CAD build for the part. Positions are in the model's coordinates, mm. Face numbers are marked on the shaded views. A direction names the side the tool comes from. Coordinates: 2 decimals unless noted, no trailing zeros. Write each loop counter-clockwise with the first axis right and the second up, starting at its lowest first coordinate (ties: lowest second). Pieces come first, ordered by that corner, then holes. Notation, with made-up numbers: (32, -17) -> (37, -17) arc R31 ccw to (37, 12) -> close; hole circle Ø4 at (81, 8). An arc over 180 degrees is marked (long way). Answer as CSV lines item,"result".
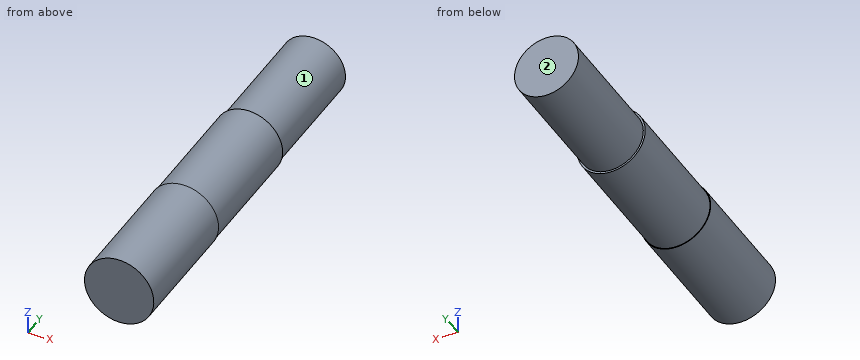
```python
from build123d import *

# Parameters (mm, degrees)
SKETCH1_R           = 4.7625
BOSS_EXTRUDE1_DEPTH = 38.1
SKETCH2_R           = 5.832464333
SKETCH2_R_2         = 3.3
CUT_EXTRUDE1_DEPTH  = 12.7
SKETCH3_R           = 5.346562202
SKETCH3_R_2         = 3.5
CUT_EXTRUDE2_DEPTH  = 12.7
SKETCH4_R           = 4.91764208
SKETCH4_R_2         = 3.571875
CUT_EXTRUDE3_DEPTH  = 12.7


with BuildPart() as part:
    # Sketch1 → Boss-Extrude1 (new body)
    with BuildSketch(Plane(origin=(0, 0, 0), x_dir=(1, 0, 0), z_dir=(0, 1, 0))):
        with Locations(Location((0, 0, 0), (0, 0, 90))):
            Circle(SKETCH1_R)
    extrude(amount=BOSS_EXTRUDE1_DEPTH)

    # Sketch2 → Cut-Extrude1 (cut)
    with BuildSketch(Plane(origin=(0, 38.1, 0), x_dir=(1, 0, 0), z_dir=(0, 1, 0))):
        Circle(SKETCH2_R)
        with Locations(Location((0, 0, 0), (0, 0, 270))):
            Circle(SKETCH2_R_2, mode=Mode.SUBTRACT)
    extrude(amount=-CUT_EXTRUDE1_DEPTH, mode=Mode.SUBTRACT)

    # Sketch3 → Cut-Extrude2 (cut)
    with BuildSketch(Plane(origin=(0, 25.4, 0), x_dir=(1, 0, 0), z_dir=(0, 1, 0))):
        Circle(SKETCH3_R)
        with Locations(Location((0, 0, 0), (0, 0, 270))):
            Circle(SKETCH3_R_2, mode=Mode.SUBTRACT)
    extrude(amount=-CUT_EXTRUDE2_DEPTH, mode=Mode.SUBTRACT)

    # Sketch4 → Cut-Extrude3 (cut)
    with BuildSketch(Plane.XZ):
        Circle(SKETCH4_R)
        with Locations(Location((0, 0, 0), (0, 0, 270))):
            Circle(SKETCH4_R_2, mode=Mode.SUBTRACT)
    extrude(amount=-CUT_EXTRUDE3_DEPTH, mode=Mode.SUBTRACT)


solid = part.part
```
Item 1: 3-axis set-ups, long thin cutter, end or side, ignore diameter. For the marked faces 1 and 2: which of +Z, -Z, +X, -X, +Y, -Y reach the whole face in a straight line?
Answer below:
face 1,"+Y"
face 2,"+Z, -Z, +X, -X, +Y"
Item 2: Saw through at A-A on z = 0. Give the cut face in (x, y), and give its area (3 significant figures).
Answer below:
outline,"(-3.57, 0) -> (3.57, 0) -> (3.57, 12.7) -> (3.5, 12.7) -> (3.5, 25.4) -> (3.3, 25.4) -> (3.3, 38.1) -> (-3.3, 38.1) -> (-3.3, 25.4) -> (-3.5, 25.4) -> (-3.5, 12.7) -> (-3.57, 12.7) -> close"
area,"263 mm2"
Item 3: Wall check: line 1 (Y direction, x = -2.5, z = -2.5); line 2 (Z direction, x = -0.75, y = 12.5); line 3 (Z direction, x = 1.5, y = 27). Give the ranges that are in metal, low to high. Write a range as from..to.
Answer below:
line 1,"y = 0..12.7"
line 2,"z = -3.49..3.49"
line 3,"z = -2.94..2.94"
Item 4: Saw through at D-D on y = 17.5. Give the cut face in (x, z).
Answer below:
outline,"circle Ø7 at (0, 0)"
Item 5: Saw through at B-B on y = 8. Give the cut face in (x, z), and give its area (3 significant figures).
Answer below:
outline,"circle Ø7.14 at (0, 0)"
area,"40.1 mm2"
Item 6: Flat gauge pin, fed straight in: pin 1 (3 mm diameter, centred on y = 22.5, z = 0, fed in from -X). Where does the tip first touch, or does it go through?
Answer below:
pin 1,"stops at x = -3.5"
Item 7: Saw through at C-C on x = 2. Give the cut face in (y, z), and give its area (3 significant figures).
Answer below:
outline,"(0, -2.96) -> (12.7, -2.96) -> (12.7, -2.87) -> (25.4, -2.87) -> (25.4, -2.62) -> (38.1, -2.62) -> (38.1, 2.62) -> (25.4, 2.62) -> (25.4, 2.87) -> (12.7, 2.87) -> (12.7, 2.96) -> (0, 2.96) -> close"
area,"215 mm2"
